```python
from build123d import *

# Parameters (mm, degrees)
F0_R     = 5
F1_DEPTH = 15
F2_R     = 11.5
F3_DEPTH = 14


with BuildPart() as f1:
    # F0 (on Top) → F1 (new body)
    with BuildSketch(Plane.XY):
        Polygon((15, 0.609152), (15, 2.061703), (14.608107, 3.460388), (12.171364, 2.891001), (11.901568, 3.853918), (14.279412, 4.633515), (13.887519, 6.032201), (13.132797, 7.273288), (10.940035, 6.06759), (10.420451, 6.922009), (12.499785, 8.314231), (11.745064, 9.555318), (10.683488, 10.546761), (8.897332, 8.794173), (8.166496, 9.476726), (9.793107, 11.378318), (8.731531, 12.369761), (7.441833, 13.038029), (6.194756, 10.868533), (5.30687, 11.328598), (6.360118, 13.598528), (5.07042, 14.266796), (3.648252, 14.562326), (3.032742, 12.136823), (2.053658, 12.340279), (2.455429, 14.810197), (1.03326, 15.105727), (-0.415904, 15.006602), (-0.354196, 12.504981), (-1.351865, 12.436738), (-1.631368, 14.923462), (-3.080532, 14.824336), (-4.449214, 14.337907), (-3.714865, 11.945701), (-4.657126, 11.610822), (-5.597175, 13.929921), (-6.965856, 13.443492), (-8.152546, 12.605835), (-6.800019, 10.500464), (-7.616989, 9.923784), (-9.147864, 11.903262), (-10.334554, 11.065605), (-11.251241, 9.938846), (-9.380847, 8.276455), (-10.011935, 7.500744), (-12.020098, 8.993793), (-12.936785, 7.867033), (-13.515483, 6.534738), (-11.265941, 5.438619), (-11.664342, 4.521408), (-14.000856, 5.417295), (-14.579554, 4.084999), (-14.777343, 2.645978), (-12.315491, 2.197426), (-12.451658, 1.20674), (-14.943235, 1.439021), (-15.141024, 0), (-14.943235, -1.439021), (-12.451658, -1.20674), (-12.315491, -2.197426), (-14.777343, -2.645978), (-14.579554, -4.084999), (-14.000856, -5.417295), (-11.664342, -4.521408), (-11.265941, -5.438619), (-13.515483, -6.534738), (-12.936785, -7.867033), (-12.020098, -8.993793), (-10.011935, -7.500744), (-9.380847, -8.276455), (-11.251241, -9.938846), (-10.334554, -11.065605), (-9.147864, -11.903262), (-7.616989, -9.923784), (-6.800019, -10.500464), (-8.152546, -12.605835), (-6.965856, -13.443492), (-5.597175, -13.929921), (-4.657126, -11.610822), (-3.714865, -11.945701), (-4.449214, -14.337907), (-3.080532, -14.824336), (-1.631368, -14.923462), (-1.351865, -12.436738), (-0.354196, -12.504981), (-0.415904, -15.006602), (1.03326, -15.105727), (2.455429, -14.810197), (2.053658, -12.340279), (3.032742, -12.136823), (3.648252, -14.562326), (5.07042, -14.266796), (6.360118, -13.598528), (5.30687, -11.328598), (6.194756, -10.868533), (7.441833, -13.038029), (8.731531, -12.369761), (9.793107, -11.378318), (8.166496, -9.476726), (8.897332, -8.794173), (10.683488, -10.546761), (11.745064, -9.555318), (12.499785, -8.314231), (10.420451, -6.922009), (10.940035, -6.06759), (13.132797, -7.273288), (13.887519, -6.032201), (14.279412, -4.633515), (11.901568, -3.853918), (12.171364, -2.891001), (14.608107, -3.460388), (15, -2.061703), (15, -0.609152), (12.5, -0.5), (12.5, 0.5), align=None)
        Circle(F0_R, mode=Mode.SUBTRACT)
    extrude(amount=F1_DEPTH)

    # F2 (on face) → F3 (cut)
    with BuildSketch(Plane(origin=(0, 0, 0), x_dir=(1, 0, 0), z_dir=(0, 0, -1))):
        Circle(F2_R)
    extrude(amount=-F3_DEPTH, mode=Mode.SUBTRACT)


solid = f1.part
```
Design review of the part built by this model. Coordinates are the model's own, in mm. A direction names the side the tool comes from. Coordinates: 2 decimals unless noted, no trailing zeros. Loops run counter-clockwise (first coordinate to the right, second up) from the corner with the lowest first, then second, coordinate; pieces in that order, holes last.
Q1. We need section A-A on x = 1.5. State the section outline as (y, z) points.
Reported:
outline: (-15.01, 0) - (-11.4, 0) - (-11.4, 14) - (-4.77, 14) - (-4.77, 15) - (-15.01, 15) - close; (4.77, 14) - (11.4, 14) - (11.4, 0) - (15.01, 0) - (15.01, 15) - (4.77, 15) - close
Q2. The part is to be moulded in two halves that separate along X. For faces 1 (the face through (9.27, 11.867, 7.395)), 2 (the face through (-4, 4, 15)), 3 (the face through (-1.5, -11.4, 6.9)), 4 (the face through (-3.77, -14.58, 7.4)), say which applies: +X half, -X half, draft (parallel to the pull), parting line (faces both ways), or undercut.
Reported:
face 1: +X half
face 2: draft
face 3: undercut
face 4: -X half
Q3. To check wall thickness, follow line 1 (Y direction, x = -9.5, z = 3.5); line 2 (X direction, y = 0, z = 10); line 3 (Y direction, x = 13, z = 6.25). State the ranges of each line that lie inside material, in increasing order.
Reported:
line 1: y = -11.65 to -8.38, -8.13 to -6.48, 6.48 to 8.13, 8.38 to 11.65
line 2: x = -15.14 to -11.5, 11.5 to 12.5
line 3: y = -7.2 to -4.21, -3.08 to -0.52, 0.52 to 3.08, 4.21 to 7.2
Q4. Tool access review of faces 5 (the face through (-5.12, 12.75, 7.4)), 6 (the face through (-1.494, -13.698, 7.395)), 7 (the face through (2.55, 12.237, 7.395)): name each direction out of +Z, -Z, +X, -X, +Y, -Y from which nothing blocks a thin tool from reaching the whole face with its end or side.
Reported:
face 5: +Z, -Z, +Y
face 6: +Z, -Z, -Y
face 7: +Z, -Z
Q5. For pin 1 (1.5 mm diameter, centred on x = -7.5, z = 6.5, fed in from +Y); pin 2 (4 mm diameter, centred on y = 7, z = 2.5, fed in from -X); pin 3 (6 mm diameter, centred on x = 7.5, z = 9.5, fed in from +Y), all flat-tipped, find the tip position at first contact; note any pin that passes through.
Reported:
pin 1: stops at y = 13.52
pin 2: stops at x = -14.18
pin 3: stops at y = 14.39
